Here's how the part is built. I have some questions about the finished solid (model axes, mm). Coordinates: 2 decimals unless noted, no trailing zeros. Write each loop counter-clockwise with the first axis right and the second up, starting at its lowest first coordinate (ties: lowest second). Pieces come first, ordered by that corner, then holes. Notation, with made-up numbers: (-4, 12) -> (43, 12) arc R15 cw to (43, 18) -> close; hole circle Ø8 at (20, 71.25). An arc over 180 degrees is marked (long way). Use a Markdown table: item, result. Add a question column.
Item 1: Imagine slicing it at B-B, the plane y = 2.25. Count the separate pieces of the cut face and the enclosed holes in it, and give its area (3 significant figures).
Item 2: If we mould it in two halves opening along X, with no side actions, what happens to faces 1 (the cylindrical face through (56.5, 3.22, 7.68)), 2 (the flat face through (-50.8, 3, 0)), 3 (the flat face through (76.2, 3, 0))? For each: pulls with the +X half, pulls with the -X half, needs draft (parallel to the pull), parting line crosses it, or undercut.
Item 3: Will this pin go through, and if not, where does the flat tip stop? pin 1 Ø23 at (x, z) = (44.45, 0) entering from -Y.
Item 4: Imagine slicing it at A-A, the plane x = 44.45. Write out the boundary of the cut face in (y, z), and give its area (3 significant figures).
Item 5: Imagine slicing it at D-D, the plane x = -38.1. Write out the boundary of the cut face in (y, z), and give its area (3 significant figures).
Item 6: If I drill on line 1 along Z through (x, y) = (-38.1, 3); line 2 along X through (y, z) = (2, 19.05); line 3 along X through (y, z) = (6, -17), over which ranges is the centre line in solid material (lowest first)? Write a range as from..to.
Item 7: Imagine slicing it at C-C, the plane z = 12.5. Write out the boundary of the cut face in (x, y).
```python
from build123d import *

# Parameters (mm, degrees)
BOSS_EXTRUDE1_DEPTH    = 6.35
F_10_CLEARANCE_HOLE1_D = 5.1054
SKETCH5_R              = 14.2875
CUT_EXTRUDE1_DEPTH     = 83.793870546


with BuildPart() as part:
    # Sketch1 → Boss-Extrude1 (new body)
    with BuildSketch(Plane(origin=(0, 0, 0), x_dir=(1, 0, 0), z_dir=(0, 1, 0))):
        Polygon((50.8, 31.75), (76.2, 31.75), (76.2, -31.75), (50.8, -31.75), (-50.8, -31.75), (-50.8, 31.75), align=None)
    extrude(amount=BOSS_EXTRUDE1_DEPTH)

    # #10 Clearance Hole1 (through all)
    with Locations(Plane(origin=(0, 6.35, 0), x_dir=(1, 0, 0), z_dir=(0, 1, 0))):
        with Locations((-38.1, 19.05), (-12.7, 19.05), (-12.7, -19.05), (-38.1, -19.05)):
            Hole(F_10_CLEARANCE_HOLE1_D / 2)

    # Sketch5 → Cut-Extrude1 (cut, through all)
    with BuildSketch(Plane(origin=(0, 6.35, 0), x_dir=(1, 0, 0), z_dir=(0, 1, 0))):
        with Locations(Location((44.45, 0, 0), (0, 0, 270))):
            Circle(SKETCH5_R)
    extrude(amount=-CUT_EXTRUDE1_DEPTH, mode=Mode.SUBTRACT)


solid = part.part
```
Ans:
| question | item | result |
|---|---|---|
| 1 | separate pieces | 1 |
| 1 | enclosed holes | 5 |
| 1 | area | 7,340 mm^2 |
| 2 | face 1 | undercut |
| 2 | face 2 | pulls with the -X half |
| 2 | face 3 | pulls with the +X half |
| 3 | pin 1 | passes through |
| 4 | outline | (0, -31.75) -> (6.35, -31.75) -> (6.35, -14.29) -> (0, -14.29) -> close; (0, 14.29) -> (6.35, 14.29) -> (6.35, 31.75) -> (0, 31.75) -> close |
| 4 | area | 222 mm^2 |
| 5 | outline | (0, -31.75) -> (6.35, -31.75) -> (6.35, -21.6) -> (0, -21.6) -> close; (0, -16.5) -> (6.35, -16.5) -> (6.35, 16.5) -> (0, 16.5) -> close; (0, 21.6) -> (6.35, 21.6) -> (6.35, 31.75) -> (0, 31.75) -> close |
| 5 | area | 338 mm^2 |
| 6 | line 1 | z = -31.75..-21.6, -16.5..16.5, 21.6..31.75 |
| 6 | line 2 | x = -50.8..-40.65, -35.55..-15.25, -10.15..76.2 |
| 6 | line 3 | x = -50.8..-39.62, -36.58..-14.22, -11.18..76.2 |
| 7 | outline | (-50.8, 0) -> (37.53, 0) -> (37.53, 6.35) -> (-50.8, 6.35) -> close; (51.37, 0) -> (76.2, 0) -> (76.2, 6.35) -> (51.37, 6.35) -> close |
